Could you check a few things on this model? Use its own coordinates, in mm. Face numbers are marked on the shaded views. A direction names the side the tool comes from. Coordinates: 2 decimals unless noted, no trailing zeros. Order: outer loops, then holes, each group sorted by start corner. A loop starts at its lowest first (then second) coordinate and runs counter-clockwise, first axis right, second up.
```python
from build123d import *

# Parameters (mm, degrees)
SKETCH1_W            = 84.8
SKETCH1_H            = 56
BOSS_EXTRUDE1_DEPTH  = 1.6
M3_CLEARANCE_SLOT1_D = 3.2
SKETCH5_W            = 50.5
SKETCH5_H            = 4.7
BOSS_EXTRUDE2_DEPTH  = 8.5
SKETCH6_W            = 21.1
SKETCH6_H            = 15.7
BOSS_EXTRUDE3_DEPTH  = 13.8
SKETCH7_W            = 17
SKETCH7_H            = 13.3
BOSS_EXTRUDE4_DEPTH  = 15.3
SKETCH8_W            = 7.2
SKETCH8_H            = 5.5
BOSS_EXTRUDE5_DEPTH  = 2.4
SKETCH9_W            = 14.8
SKETCH9_H            = 11.4
BOSS_EXTRUDE6_DEPTH  = 6.3
SKETCH10_W           = 6.8
SKETCH10_H           = 11.8
BOSS_EXTRUDE7_DEPTH  = 6
SKETCH11_R           = 2.85
BOSS_EXTRUDE8_DEPTH  = 2.2


with BuildPart() as part:
    # Sketch1 → Boss-Extrude1 (new body)
    with BuildSketch(Plane(origin=(0, 0, 0), x_dir=(1, 0, 0), z_dir=(0, 1, 0))):
        with Locations((42.4, 28)):
            Rectangle(SKETCH1_W, SKETCH1_H)
    extrude(amount=BOSS_EXTRUDE1_DEPTH)

    # M3 Clearance Slot1 (through all)
    with Locations(Plane(origin=(0, 1.6, 0), x_dir=(1, 0, 0), z_dir=(0, 1, 0))):
        with Locations((81.6, 3.2), (81.6, 52.8), (23, 52.8), (23, 3.2)):
            Hole(M3_CLEARANCE_SLOT1_D / 2)

    # Sketch5 → Boss-Extrude2 (add)
    with BuildSketch(Plane(origin=(0, 1.6, 0), x_dir=(1, 0, 0), z_dir=(0, 1, 0))):
        with Locations((52.55, 3.55)):
            Rectangle(SKETCH5_W, SKETCH5_H)
    extrude(amount=BOSS_EXTRUDE2_DEPTH)

    # Sketch6 → Boss-Extrude3 (add)
    with BuildSketch(Plane(origin=(0, 1.6, 0), x_dir=(1, 0, 0), z_dir=(0, 1, 0))):
        with Locations((8.25, 45.85)):
            Rectangle(SKETCH6_W, SKETCH6_H)
    extrude(amount=BOSS_EXTRUDE3_DEPTH)

    # Sketch7 → Boss-Extrude4 (add)
    with BuildSketch(Plane(origin=(0, 1.6, 0), x_dir=(1, 0, 0), z_dir=(0, 1, 0))):
        with Locations((6.2, 27.15)):
            Rectangle(SKETCH7_W, SKETCH7_H)
        with Locations((6.2, 9.05)):
            Rectangle(SKETCH7_W, SKETCH7_H)
    extrude(amount=BOSS_EXTRUDE4_DEPTH)

    # Sketch8 → Boss-Extrude5 (add)
    with BuildSketch(Plane(origin=(0, 1.6, 0), x_dir=(1, 0, 0), z_dir=(0, 1, 0))):
        with Locations((74.3, 54.45)):
            Rectangle(SKETCH8_W, SKETCH8_H)
    extrude(amount=BOSS_EXTRUDE5_DEPTH)

    # Sketch9 → Boss-Extrude6 (add)
    with BuildSketch(Plane(origin=(0, 1.6, 0), x_dir=(1, 0, 0), z_dir=(0, 1, 0))):
        with Locations((52.4, 51.7)):
            Rectangle(SKETCH9_W, SKETCH9_H)
    extrude(amount=BOSS_EXTRUDE6_DEPTH)

    # Sketch10 → Boss-Extrude7 (add)
    with BuildSketch(Plane(origin=(0, 1.6, 0), x_dir=(1, 0, 0), z_dir=(0, 1, 0))):
        with Locations((33.722871629, 50.09)):
            Rectangle(SKETCH10_W, SKETCH10_H)
    extrude(amount=BOSS_EXTRUDE7_DEPTH)

    # Sketch11 → Boss-Extrude8 (add)
    with BuildSketch(Plane(origin=(0, 0, -55.99), x_dir=(-1, 0, 0), z_dir=(0, 0, -1))):
        with Locations(Location((-33.722871629, 4.6, 0), (0, 0, 180))):
            Circle(SKETCH11_R)
    extrude(amount=BOSS_EXTRUDE8_DEPTH)


solid = part.part
```
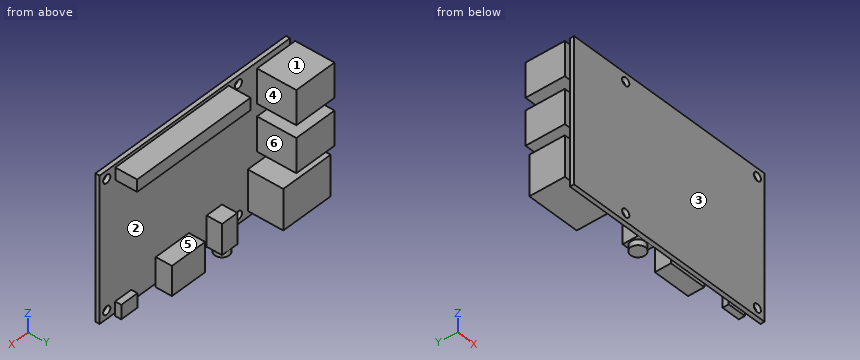
Item 1: I need wall thicknesses on line 1 (X direction, y = 0.9, z = -52.8); line 2 (Z direction, x = 11, y = 2.75); line 3 (Z direction, x = 3, y = 15.5). Which ranges of each line are inside material? Lowest first, please.
Item 2: Thinking about a two-plate mould opening in Z: for the marked faces 1, 2 and 3, which applies, +Z half, -Z half, draft (parallel to the pull), parting line (faces both ways), or undercut?
Item 3: Which directions (+Z, -Z, +X, -X, +Y, -Y) give clear straight access to the entire face, cutting with the end or side of a thin tool? Please do the marked faces 4, 5 and 6.
Item 4: Suppose I cut it at B-B (y = 6.5). List the corners of the cut face in (x, z) for me.
Item 5: For pin 1 Ø1.8 at (x, z) = (-1.5, -29) entering from -Y; pin 2 Ø1.5 at (x, y) = (51, 10.5) entering from -Z; pin 3 Ø2.5 at (y, z) = (4, -3.5) entering from +X, each with a flat end and sliding along its axis, tell me the tip position at first contact or that it passes through.
Item 6: Suppose I cut it at C-C (z = -52.8). List the corners of the cut face in (x, y) for me.
Item 7: Suppose I cut it at A-A (x = 81.6). List the corners of the cut face in (y, z) for me.
Item 8: Suppose I cut it at D-D (z = -23). List the corners of the cut face in (x, y) for me.
Geometry results:
1. line 1: x = 0 to 21.4, 24.6 to 80, 83.2 to 84.8
1. line 2: z = -53.7 to -38, -33.8 to -20.5, -15.7 to -2.4
1. line 3: z = -33.8 to -20.5, -15.7 to -2.4
2. face 1: +Z half
2. face 2: undercut
2. face 3: draft
3. face 4: +Z, +Y
3. face 5: +X, +Y
3. face 6: +Z, +X, +Y
4. outline: (-2.3, -53.7) - (18.8, -53.7) - (18.8, -38) - (-2.3, -38) - close; (-2.3, -33.8) - (14.7, -33.8) - (14.7, -20.5) - (-2.3, -20.5) - close; (-2.3, -15.7) - (14.7, -15.7) - (14.7, -2.4) - (-2.3, -2.4) - close; (27.3, -5.9) - (77.8, -5.9) - (77.8, -1.2) - (27.3, -1.2) - close; (30.32, -55.99) - (31.6, -55.99) - (31.6, -58.19) - (35.85, -58.19) - (35.85, -55.99) - (37.12, -55.99) - (37.12, -44.19) - (30.32, -44.19) - close; (45, -57.4) - (59.8, -57.4) - (59.8, -46) - (45, -46) - close
5. pin 1: stops at y = 1.6
5. pin 2: stops at z = -5.9
5. pin 3: stops at x = 77.8
6. outline: (-2.3, 1.6) - (0, 1.6) - (0, 0) - (21.4, 0) - (21.4, 1.6) - (18.8, 1.6) - (18.8, 15.4) - (-2.3, 15.4) - close; (24.6, 0) - (80, 0) - (80, 1.6) - (77.9, 1.6) - (77.9, 4) - (70.7, 4) - (70.7, 1.6) - (59.8, 1.6) - (59.8, 7.9) - (45, 7.9) - (45, 1.6) - (37.12, 1.6) - (37.12, 7.6) - (30.32, 7.6) - (30.32, 1.6) - (24.6, 1.6) - close; (83.2, 0) - (84.8, 0) - (84.8, 1.6) - (83.2, 1.6) - close
7. outline: (0, -56) - (1.6, -56) - (1.6, -54.4) - (0, -54.4) - close; (0, -51.2) - (1.6, -51.2) - (1.6, -4.8) - (0, -4.8) - close; (0, -1.6) - (1.6, -1.6) - (1.6, 0) - (0, 0) - close
8. outline: (-2.3, 1.6) - (0, 1.6) - (0, 0) - (84.8, 0) - (84.8, 1.6) - (14.7, 1.6) - (14.7, 16.9) - (-2.3, 16.9) - close
